Read the model definition and answer for the solid it produces. Units are mm, in the model's axes. A direction names the side the tool comes from. Round coordinates to 2 decimals unless told otherwise and drop trailing zeros. Write each loop counter-clockwise with the first axis right and the second up, starting at its lowest first coordinate (ties: lowest second). Pieces come first, ordered by that corner, then holes. Notation, with made-up numbers: (33, 42.5) - (71, 42.5) arc R12 cw to (71, 48.5) - close; hole circle Ø10 at (6, 44.5). An arc over 180 degrees is marked (long way). Use one line per item in the form item = value. Start each with the question number.
1) For faces 4 (the face through (-13.82, 7.53, 18.9)), 5 (the face through (16, 0, 2)), 6 (the face through (-16, 0, 2)), 7 (the face through (0, 6, 0)), determine the directions among +Z, -Z, +X, -X, +Y, -Y from which every point of the face is accessible in a straight line to the end or side of a thin tool.
2) The part is cut by section B-B, the plane y = 2. Give the vertices of the cut face in (x, z).
3) The part is cut by section D-D, the plane x = 10. Give the vertices of the cut face in (y, z).
4) The part is cut by section C-C, the plane y = 12. Give the vertices of the cut face in (x, z).
5) The part is cut by section A-A, the plane x = 0. Give the vertices of the cut face in (y, z).
6) Consider line 1 along Y through (x, z) = (0, -1); line 2 along Z through (x, y) = (5, 10); line 3 along X through (y, z) = (9.75, 2). Determine where each line is inside the solid, lowest interval first. Write a range as from..to.
7) Each of these flat-tipped pins is pushed along its axis until it touches: pin 1 (2.5 mm diameter, centred on x = 15, z = 3.5, fed in from -Y); pin 2 (5 mm diameter, centred on x = 0, y = 0, fed in from +Z); pin 3 (4 mm diameter, centred on x = 2.5, z = 27.5, fed in from -Y); pin 4 (12 mm diameter, centred on y = 9.5, z = 36, fed in from -X). Where does it stop, or does it pass through?
8) For a pull along Z with two mould halves and no side action, classify faces 1 (the face through (-0.1, -7.5, -1)), 2 (the face through (0, 5, 40.1)), 3 (the face through (0, 6, 38.1)) as released by +Z, released by -Z, zero draft, split by the parting line, or undercut.
Autodesk Inventor part; units mm, degrees
ref_plane "YZ Plane" through (0, 0, 0) normal (1, 0, 0) x (0, 1, 0)
ref_plane "XZ Plane" through (0, 0, 0) normal (0, 1, 0) x (-1, 0, 0)
ref_plane "XY Plane" through (0, 0, 0) normal (0, 0, 1) x (1, 0, 0)
sketch "Sketch1" plane through (0, 0, 0) normal (0, 0, 1) x (1, 0, 0)
  circle A0 centre (0, 0) radius 4.1
  circle A1 centre (0, 0) radius 15
  circle A2 centre (0, 0) radius 16.5
  line L0 (-16.5, 0) -> (16.5, 0)
  circle A3 centre (0, 0) radius 7.5
  line L1 (-7.5, 0) -> (-14.3434, 8.1557)
  line L2 (7.5, 0) -> (14.3434, 8.1557)
  point P0 (-15, 0)
  point P1 (15, 0)
  point P2 (13.3077, 6.9213)
  point P3 (-13.3077, 6.9213)
  dimension "d0" = 8.2
  dimension "d1" = 30
  dimension "d2" = 33
  dimension "d5" = 15
  dimension "d6" = 50
extrude "Extrusion1" add sketch "Sketch1" along normal blind 19.05 contours A1 L1 A2 L2
extrude "Extrusion2" add sketch "Sketch1" against normal blind 2 contours L0 A3 A0 | A0 L0 A3 | L2 A1 L0 | A3 L1 A1 L2 | L0 A1 L1 | A1 L2 A2 L0 | A1 L1 A2 L2 | L0 A2 L1 A1
extrude "Extrusion3" add sketch "Sketch1" along normal blind 8 contours A1 L2 A2 L0 | L0 A2 L1 A1
mirror "Mirror1" about plane through (0, 11.7107, 19.05) normal (0, 0, 1)
fillet "Fillet1" radius 5 4 edges at (-7.5, 0, -1) (7.5, 0, -1) (7.5, 0, 39.1) (-7.5, 0, 39.1)
properties part number "pulley_bearing_base_cover"
Geometry results:
q1.face_4 = -X, -Y
q1.face_5 = +Z, -Z, +X, -Y
q1.face_6 = +Z, -Z, -X, -Y
q1.face_7 = -Y
q2.outline = (-16.38, -2) - (-3.58, -2) - (-3.58, 0) - (-14.87, 0) - (-14.87, 8) - (-16.38, 8) - close; (-16.38, 30.1) - (-14.87, 30.1) - (-14.87, 38.1) - (-3.58, 38.1) - (-3.58, 40.1) - (-16.38, 40.1) - close; (3.58, -2) - (16.38, -2) - (16.38, 8) - (14.87, 8) - (14.87, 0) - (3.58, 0) - close; (3.58, 38.1) - (14.87, 38.1) - (14.87, 30.1) - (16.38, 30.1) - (16.38, 40.1) - (3.58, 40.1) - close
q3.outline = (-0.22, -2) - (13.12, -2) - (13.12, 40.1) - (-0.22, 40.1) - (-0.22, 38.1) - (11.18, 38.1) - (11.18, 0) - (-0.22, 0) - close
q4.outline = (-11.32, -2) - (11.32, -2) - (11.32, 40.1) - (-11.32, 40.1) - close; hole (-9, 0) - (9, 0) - (9, 38.1) - (-9, 38.1) - close
q5.outline = (-7.5, -2) - (-4.1, -2) - (-4.1, 0) - (-7.5, 0) - close; (-7.5, 38.1) - (-4.1, 38.1) - (-4.1, 40.1) - (-7.5, 40.1) - close; (4.1, -2) - (16.5, -2) - (16.5, 40.1) - (4.1, 40.1) - (4.1, 38.1) - (15, 38.1) - (15, 0) - (4.1, 0) - close
q6.line_1 = -7.5..-4.1, 4.1..16.5
q6.line_2 = -2..0, 38.1..40.1
q6.line_3 = -13.31..-11.4, 11.4..13.31
q7.pin_1 = 0
q7.pin_2 = through
q7.pin_3 = 14.31
q7.pin_4 = -16.12
q8.face_1 = zero draft
q8.face_2 = released by +Z
q8.face_3 = undercut
